Autodesk Inventor part; units mm, degrees
ref_plane "YZ Plane" through (0, 0, 0) normal (1, 0, 0) x (0, 1, 0)
ref_plane "XZ Plane" through (0, 0, 0) normal (0, 1, 0) x (-1, 0, 0)
ref_plane "XY Plane" through (0, 0, 0) normal (0, 0, 1) x (1, 0, 0)
sketch "Sketch1" plane through (0, 0, 0) normal (0, 0, 1) x (1, 0, 0)
  line L0 (-15, 15) -> (15, 15)
  line L1 (15, 15) -> (15, -15)
  line L2 (15, -15) -> (-15, -15)
  line L3 (-15, -15) -> (-15, 15)
  point P0 (0, 0)
  dimension "d0" = 30
  dimension "d1" = 30
  dimension "d2" = 15
  dimension "d3" = 15
extrude "Extrusion1" add sketch "Sketch1" along normal blind 18
sketch "Sketch2" plane through (-15, 15, 0) normal (0, 1, 0) x (1, 0, 0)
  circle A0 centre (6.5, -3) radius 1.5
  circle A1 centre (23.5, -3) radius 1.5
  circle A2 centre (15, -15) radius 1.5
  circle A3 centre (6, -12) radius 2.5
  circle A4 centre (24, -12) radius 2.5
  line L0 (0, 0) -> (30, 0)
  line L1 (15, 0) -> (15, -28.1045) construction
  line L2 (30, -18) -> (0, -18) construction
  line L3 (6, -12) -> (24, -12) construction
  dimension "d6" = 3
  dimension "d7" = 3
  dimension "d8" = 3
  dimension "d9" = 5
  dimension "d10" = 5
  dimension "d11" = 17
  dimension "d12" = 3
  dimension "d13" = 3
  dimension "d14" = 8.5
  dimension "d15" = 18
  dimension "d16" = 9
  dimension "d17" = 3
  dimension "d18" = 6
  dimension "d19" = 6
  dimension "d20" = 0
  dimension "d51" = 3
  dimension "d52" = 9
extrude "Extrusion2" cut sketch "Sketch2" against normal blind 10
thread "Thread3"
thread "Thread4"
thread "Thread5"
sketch "Sketch3" plane through (-9, 5, 12) normal (0, 1, 0) x (1, 0, 0)
  circle A0 centre (0, 0) radius 1
  point P0 (9, 12)
  dimension "d23" = 2
extrude "Extrusion3" cut sketch "Sketch3" against normal through all
sketch "Sketch4" plane through (9, 5, 12) normal (0, 1, 0) x (1, 0, 0)
  circle A0 centre (0, 0) radius 1
  point P0 (-9, 12)
  dimension "d26" = 2
extrude "Extrusion4" cut sketch "Sketch4" against normal through all
sketch "Sketch5" plane through (-15, -15, 0) normal (0, -1, 0) x (1, 0, 0)
  circle A0 centre (6, 12) radius 1
  circle A1 centre (6, 12) radius 3.5
  circle A2 centre (24, 12) radius 1
  circle A3 centre (24, 12) radius 3.5
  point P0 (15, 0)
  dimension "d29" = 7
  dimension "d30" = 7
extrude "Extrusion5" cut sketch "Sketch5" against normal blind 15
sketch "Sketch6" plane through (0, 0, 0) normal (0, 0, -1) x (-1, 0, 0)
  line L0 (15, 15) -> (15, -15)
  line L1 (-15, -13.25) -> (15, -13.25)
  line L2 (15, -13.25) -> (15, -10.75)
  line L3 (15, -10.75) -> (-15, -10.75)
  line L4 (-15, -10.75) -> (-15, -13.25)
  line L5 (-15, -15) -> (15, -15)
  line L6 (-15, 10.75) -> (15, 10.75)
  line L7 (15, 10.75) -> (15, 13.25)
  line L8 (15, 13.25) -> (-15, 13.25)
  line L9 (-15, 13.25) -> (-15, 10.75)
  line L10 (15, 15) -> (-15, 15)
  line L11 (-15, -8.75) -> (15, -8.75)
  line L12 (15, -8.75) -> (15, -6.75)
  line L13 (15, -6.75) -> (-15, -6.75)
  line L14 (-15, -6.75) -> (-15, -8.75)
  line L15 (15, -2.75) -> (-15, -2.75)
  line L16 (-15, -2.75) -> (-15, -4.75)
  line L17 (-15, -4.75) -> (15, -4.75)
  line L18 (15, -4.75) -> (15, -2.75)
  line L19 (15, 1.25) -> (-15, 1.25)
  line L20 (-15, 1.25) -> (-15, -0.75)
  line L21 (-15, -0.75) -> (15, -0.75)
  line L22 (15, -0.75) -> (15, 1.25)
  line L23 (15, 5.25) -> (-15, 5.25)
  line L24 (-15, 5.25) -> (-15, 3.25)
  line L25 (-15, 3.25) -> (15, 3.25)
  line L26 (15, 3.25) -> (15, 5.25)
  line L27 (15, 9.25) -> (-15, 9.25)
  line L28 (-15, 9.25) -> (-15, 7.25)
  line L29 (-15, 7.25) -> (15, 7.25)
  line L30 (15, 7.25) -> (15, 9.25)
  point P0 (0, 0)
  dimension "d33" = 30
  dimension "d34" = 30
  dimension "d35" = 2.5
  dimension "d36" = 1.75
  dimension "d37" = 2.5
  dimension "d38" = 30
  dimension "d39" = 1.75
  dimension "d40" = 2
  dimension "d41" = 2
  dimension "d44" = 4
extrude "Extrusion6" cut sketch "Sketch6" against normal blind 6
thread "Thread1"
thread "Thread2"
sketch "Sketch7" plane through (0, 0, 18) normal (0, 0, 1) x (1, 0, 0)
  circle A0 centre (-9, -12) radius 1.5
  circle A1 centre (9, -12) radius 1.5
  circle A2 centre (9, -5) radius 1.5
  circle A3 centre (-9, -5) radius 1.5
  line L0 (-5.5, -15) -> (-12.5, -15)
  line L1 (-15, -15) -> (15, -15)
  point P0 (0, 0)
  dimension "d63" = 3
  dimension "d64" = 3
  dimension "d65" = 3
  dimension "d66" = 3
  dimension "d67" = 18
  dimension "d68" = 18
  dimension "d69" = 9
  dimension "d70" = 9
  dimension "d71" = 3
  dimension "d72" = 3
  dimension "d73" = 7
  dimension "d74" = 7
extrude "Extrusion7" cut sketch "Sketch7" against normal up to next
thread "Thread6"
thread "Thread7"
thread "Thread8"
thread "Thread9"
equation "\"d13\" = d12"
equation "\"d14\" = 0.5 * d11"
equation "\"d16\" = 0.5 * d15"
equation "\"d19\" = d18"
equation "\"d34\" = d33"
equation "\"d37\" = d35"
equation "\"d38\" = d33"
equation "\"d39\" = d36"
equation "\"d41\" = d40"
equation "\"d68\" = d67"
equation "\"d74\" = d73"
properties part number "nozzel heat sink"
Build history of the part. All positions in model axes, mm. A direction names the side the tool comes from. Give positions to 0.01 mm unless a question says otherwise; leave off trailing zeros. Order: outer loops, then holes, each group sorted by start corner. A loop starts at its lowest first (then second) coordinate and runs counter-clockwise, first axis right, second up. Notation, with made-up numbers: M 67.5,-9.75 L 78.5,-9.75 A5 cw 78.5,-4.75 Z; hole C 46,-20 d2. An arc over 180 degrees is marked long. Return JSON: item names as keys, results as strings.
Q1. Wall check: probe 1 along X at (y, z) = (14.6, 3); probe 2 along X at (y, z) = (2.7, 12); probe 3 along Z at (x, y) = (9, -9.75). Give the ranges that are in metal, low to high. Write a range as from..to.
Answer list:
{"probe 1": "x = -15..-10, -7..7, 10..15", "probe 2": "x = -15..-10, -8..8, 10..15", "probe 3": "z = 0..8.5, 15.5..18"}
Q2. 3-axis set-ups, long thin cutter, end or side, ignore diameter. For faces 1 (the face through (10, 5, 13)), 2 (the face through (7.5, -4.93, 16.6)), 3 (the face through (0, -2.75, 3)), 4 (the face through (10, 0, 11)), 5 (the face through (15, 0, 11)): which of +Z, -Z, +X, -X, +Y, -Y reach the whole face in a straight line?
Answer list:
{"face 1": "+Y", "face 2": "+Z", "face 3": "-Z, +X, -X", "face 4": "-Y", "face 5": "+Z, -Z, +X, +Y, -Y"}
Q3. Band-saw the part on B-B (y = -7.5). Give the cut face in (x, z).
Answer list:
{"outline": "M -15,6 L 15,6 L 15,18 L -15,18 Z; hole C -9,12 d7; hole C 9,12 d7"}
Q4. Band-saw the part on A-A (z = 12). Give the cut face in (x, y).
Answer list:
{"outline": "M -15,-15 L -12.5,-15 L -12.5,0 L -10,0 L -10,5 L -11.5,5 L -11.5,15 L -15,15 Z; M -8,0 L -5.5,0 L -5.5,-15 L 5.5,-15 L 5.5,0 L 8,0 L 8,5 L 6.5,5 L 6.5,15 L -6.5,15 L -6.5,5 L -8,5 Z; M 10,0 L 12.5,0 L 12.5,-15 L 15,-15 L 15,15 L 11.5,15 L 11.5,5 L 10,5 Z"}
Q5. Band-saw the part on C-C (y = 6.5). Give the cut face in (x, z), then the cut area to 3 significant figures.
Answer list:
{"outline": "M -15,0 L 15,0 L 15,18 L -15,18 Z; hole C -9,12 d5; hole C -8.5,3 d3; hole C 0,15 d3; hole C 9,12 d5; hole C 8.5,3 d3", "area": "480 mm^2"}
Q6. Flat gauge pins, fed straight in: pin 1 (1 mm diameter, centred on x = -4, y = 8, fed in from -Z); pin 2 (2 mm diameter, centred on x = -10.5, z = 11, fed in from -Y); pin 3 (1.6 mm diameter, centred on x = 9, z = 12, fed in from +Y); pin 4 (12 mm diameter, centred on x = 7.5, y = -5.5, fed in from -Z). Where does each tip first touch, or does it go through?
Answer list:
{"pin 1": "stops at z = 6", "pin 2": "stops at y = 0", "pin 3": "passes through", "pin 4": "stops at z = 0"}
Q7. Band-saw the part on D-D (z = 3). Count the separate pieces of the cut face and the enclosed holes in it, then the cut area to 4 significant figures.
Answer list:
{"separate pieces": "14", "enclosed holes": "0", "area": "418.5 mm^2"}
Q8. Two-plate mould, pull along Z, no slides. Class faces 6 (the face through (0, 0, 18)), 7 (the face through (-8, 0, 11)), 8 (the face through (0, 10.75, 3)): pulls with the +Z half, pulls with the -Z half, needs draft (parallel to the pull), parting line crosses it, or undercut.
Answer list:
{"face 6": "pulls with the +Z half", "face 7": "undercut", "face 8": "needs draft"}
